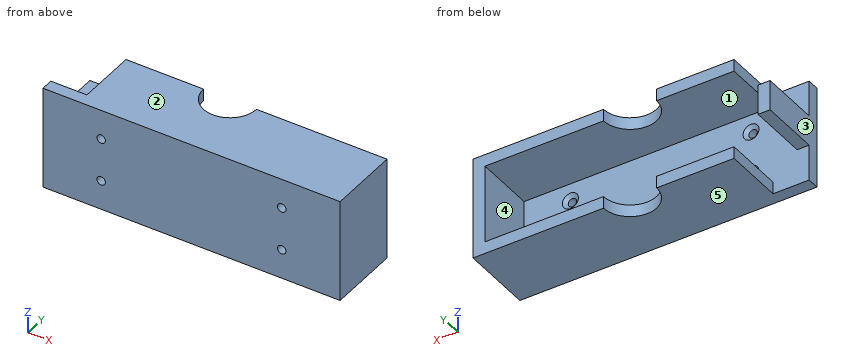
```python
from build123d import *

# Parameters (mm, degrees)
BOSS_EXTRUDE1_DEPTH                               = 38.1
SKETCH1_W                                         = 6.35
SKETCH1_H                                         = 16.002
BOSS_EXTRUDE1_2_DEPTH                             = 38.1
SKETCH1_4_W                                       = 144.018
SKETCH1_4_H                                       = 41.402
BOSS_EXTRUDE2_DEPTH                               = 6.35
SKETCH1_5_W                                       = 131.318
SKETCH1_5_H                                       = 6.35
BOSS_EXTRUDE3_DEPTH                               = 38.1
CSK_FOR_8_FLAT_HEAD_MACHINE_SCREW_100_D           = 4.4958
CSK_FOR_8_FLAT_HEAD_MACHINE_SCREW_100_CSINK_D     = 8.4328
CSK_FOR_8_FLAT_HEAD_MACHINE_SCREW_100_CSINK_ANGLE = 100
BOSS_EXTRUDE6_DEPTH                               = 6.35
CUT_EXTRUDE3_DEPTH                                = 105.525006773
CUT_EXTRUDE3_DEPTH_BACK                           = 105.525006773
BOSS_EXTRUDE7_DEPTH                               = 6.35


with BuildPart() as part:
    # Sketch1 → Boss-Extrude1 (new body)
    with BuildSketch(Plane(origin=(0, 0, 0), x_dir=(1, 0, 0), z_dir=(0, 1, 0))):
        Polygon((74.562549316, 16.479821782), (74.562549316, 10.129821782), (74.562549316, -31.272178218), (74.562549316, -37.622178218), (80.912549316, -37.622178218), (80.912549316, 16.479821782), align=None)
    extrude(amount=BOSS_EXTRUDE1_DEPTH)



with BuildPart() as body_2:
    # Sketch1 → Boss-Extrude1 2 (new body)
    with BuildSketch(Plane(origin=(0, 0, 0), x_dir=(1, 0, 0), z_dir=(0, 1, 0))):
        with Locations((-72.630450684, -10.571178218)):
            Rectangle(SKETCH1_W, SKETCH1_H)
    extrude(amount=BOSS_EXTRUDE1_2_DEPTH)


with BuildPart() as part_1:
    add(part.part)

    add(body_2.part)  # Boss-Extrude2 merges body 2
    # Sketch1_4 → Boss-Extrude2 (add)
    with BuildSketch(Plane(origin=(0, 0, 0), x_dir=(1, 0, 0), z_dir=(0, 1, 0))):
        with Locations((2.553549316, -10.571178218)):
            Rectangle(SKETCH1_4_W, SKETCH1_4_H)
    extrude(amount=BOSS_EXTRUDE2_DEPTH)

    # Sketch1_5 → Boss-Extrude3 (add)
    with BuildSketch(Plane(origin=(0, 0, 0), x_dir=(1, 0, 0), z_dir=(0, 1, 0))):
        with Locations((8.903549316, 13.304821782)):
            Rectangle(SKETCH1_5_W, SKETCH1_5_H)
        with Locations((8.903549316, -34.447178218)):
            Rectangle(SKETCH1_5_W, SKETCH1_5_H)
    extrude(amount=BOSS_EXTRUDE3_DEPTH)

    # CSK for _8 Flat Head Machine Screw _100 (through all)
    with Locations(Plane(origin=(0, 6.35, 0), x_dir=(1, 0, 0), z_dir=(0, 1, 0))):
        with Locations((-45.134950684, -21.937678218), (-45.134950684, 0.922321782), (50.115049316, 0.858821782), (50.115049316, -22.001178218)):
            CounterSinkHole(CSK_FOR_8_FLAT_HEAD_MACHINE_SCREW_100_D / 2, CSK_FOR_8_FLAT_HEAD_MACHINE_SCREW_100_CSINK_D / 2, counter_sink_angle=CSK_FOR_8_FLAT_HEAD_MACHINE_SCREW_100_CSINK_ANGLE)

    # Sketch1_8 → Boss-Extrude6 (add)
    with BuildSketch(Plane(origin=(0, 0, 0), x_dir=(1, 0, 0), z_dir=(0, 1, 0))):
        Polygon((-69.455450684, -31.272178218), (-69.455450684, -18.572178218), (-75.805450684, -18.572178218), (-75.805450684, -31.272178218), (-75.805450684, -37.622178218), (-56.755450684, -37.622178218), (-56.755450684, -31.272178218), align=None)
    extrude(amount=BOSS_EXTRUDE6_DEPTH)

    # Sketch11 → Cut-Extrude3 (cut, two sides: drawn at the far end of the back side and taken through both)
    with BuildSketch(Plane.XY.offset(37.622178218).offset(-CUT_EXTRUDE3_DEPTH_BACK)):
        with BuildLine():
            Line((-15.886355633, 256.15420447), (-15.886355633, 38.1))
            ThreePointArc((-15.886355633, 38.1), (-1.903903158, 24.117547525), (12.078549316, 38.1))
            Line((12.078549316, 38.1), (12.078549316, 256.15420447))
            Line((12.078549316, 256.15420447), (12.078549316, 692.262613411))
            Line((12.078549316, 692.262613411), (-15.886355633, 692.262613411))
            Line((-15.886355633, 692.262613411), (-15.886355633, 256.15420447))
        make_face()
    extrude(amount=CUT_EXTRUDE3_DEPTH + CUT_EXTRUDE3_DEPTH_BACK, mode=Mode.SUBTRACT)

    # Sketch1_9 → Boss-Extrude7 (add)
    with BuildSketch(Plane(origin=(0, 0, 0), x_dir=(1, 0, 0), z_dir=(0, 1, 0))):
        Polygon((-69.455450684, -2.570178218), (-69.455450684, 10.129821782), (-56.755450684, 10.129821782), (-56.755450684, 16.479821782), (-69.455450684, 16.479821782), (-75.805450684, 16.479821782), (-75.805450684, 10.129821782), (-75.805450684, -2.570178218), align=None)
    extrude(amount=BOSS_EXTRUDE7_DEPTH)


solid = part_1.part
```
Design review of the part built by this model. Coordinates are the model's own, in mm. Face numbers are marked on the shaded views. A direction names the side the tool comes from. Round coordinates to 2 decimals unless told otherwise and drop trailing zeros. Write each loop counter-clockwise with the first axis right and the second up, starting at its lowest first coordinate (ties: lowest second). Pieces come first, ordered by that corner, then holes.
Item 1: For the marked faces 1 and 2, list the 3-axis set-ups (+Z, -Z, +X, -X, +Y, -Y) from which the entire face can be reached by the end or side of a thin tool; tool diameter is ignored.
Item 2: We need section B-B on z = 34.5. Write out the cut boundary in (x, y).
Item 3: We need section A-A on y = 18.5. Write out the cut boundary in (x, z), and give its area (3 significant figures).
Item 4: We need section D-D on x = 8. Write out the cut boundary in (y, z).
Item 5: We need section C-C on y = 26. Write out the cut boundary in (x, z), and give its area (3 significant figures).
Item 6: Clearance check with flat-ended pins moving along their axes: pin 1 Ø3 at (x, z) = (34, 32) entering from -Y; pin 2 Ø16 at (x, z) = (3.5, 1.5) entering from +Y; pin 3 Ø6 at (x, z) = (50.12, -0.86) entering from +Y; pin 4 Ø3.5 at (x, z) = (50.12, 22) entering from -Y. State where each tip first meets the part, or that it passes through.
Item 7: The part is to be moulded in two halves that separate along Z. For the marked faces 3, 4 and 5, say which applies: +Z half, -Z half, draft (parallel to the pull), parting line (faces both ways), or undercut.
Item 8: For probe 1 along Z at (x, y) = (61, 23); probe 2 along X at (y, z) = (27, 6); probe 3 along Y at (x, z) = (-66, 19.5), list the stretches that pass through material, from the lowest coordinate up.
Returned:
1. face 1: -X, +Y
1. face 2: +Z, +X, -X, +Y, -Y
2. outline: (-75.81, 0) - (80.91, 0) - (80.91, 38.1) - (12.08, 38.1) arc R13.98 cw to (-15.89, 38.1) - (-56.76, 38.1) - (-56.76, 6.35) - (-75.81, 6.35) - close
3. outline: (-75.81, 2.57) - (-69.46, 2.57) - (-69.46, 18.57) - (-75.81, 18.57) - close; (-56.76, -16.48) - (80.91, -16.48) - (80.91, 37.62) - (-56.76, 37.62) - (-56.76, 31.27) - (74.56, 31.27) - (74.56, -10.13) - (-56.76, -10.13) - close
3. area: 2,110 mm2
4. outline: (0, -16.48) - (28.23, -16.48) - (28.23, -10.13) - (6.35, -10.13) - (6.35, 31.27) - (28.23, 31.27) - (28.23, 37.62) - (0, 37.62) - close
5. outline: (-75.81, 2.57) - (-69.46, 2.57) - (-69.46, 18.57) - (-75.81, 18.57) - close; (-56.76, -16.48) - (-8.91, -16.48) - (-8.91, -10.13) - (-56.76, -10.13) - close; (-56.76, 31.27) - (-8.91, 31.27) - (-8.91, 37.62) - (-56.76, 37.62) - close; (5.1, -16.48) - (80.91, -16.48) - (80.91, 37.62) - (5.1, 37.62) - (5.1, 31.27) - (74.56, 31.27) - (74.56, -10.13) - (5.1, -10.13) - close
5. area: 1,930 mm2
6. pin 1: stops at y = 0
6. pin 2: stops at y = 6.35
6. pin 3: stops at y = 5.33
6. pin 4: passes through
7. face 3: draft
7. face 4: undercut
7. face 5: -Z half
8. probe 1: z = -16.48 to -10.13, 31.27 to 37.62
8. probe 2: x = -75.81 to -69.46, 74.56 to 80.91
8. probe 3: y = 0 to 6.35
